```python
from build123d import *

# Parameters (mm, degrees)
RESSALTO_EXTRUS_O1_DEPTH = 10


with BuildPart() as part:
    # Esboço1 → Ressalto-extrusão1 (new body)
    with BuildSketch(Plane.XY):
        with BuildLine():
            Line((0, 14), (0, 20))
            Line((0, 20), (0, 40))
            ThreePointArc((0, 40), (-2.5, 42.5), (-5, 40))
            Line((-5, 40), (-4.923076923, 39.384615385))
            Line((-4.923076923, 39.384615385), (-3.069859681, 24.558877449))
            ThreePointArc((-3.069859681, 24.558877449), (-23.734852986, -7.015643501), (10.775337309, -22.281261317))
            Line((10.775337309, -22.281261317), (6.095140296, -12.603541755))
            ThreePointArc((6.095140296, -12.603541755), (-13.646420494, -3.126532858), (0, 14))
        make_face()
    extrude(amount=RESSALTO_EXTRUS_O1_DEPTH)


solid = part.part
```
Model file for the job. Use its own axes, mm. Coordinates: 2 decimals unless noted, no trailing zeros. Order: outer loops, then holes, each group sorted by start corner. A loop starts at its lowest first (then second) coordinate and runs counter-clockwise, first axis right, second up. Notation, with made-up numbers: (-23.5, -32.5) -> (13.5, -32.5) arc R11 ccw to (13.5, -18.5) -> close; hole circle Ø7 at (36, 35). An arc over 180 degrees is marked (long way). Answer as a JSON object with one key per item and string values. Group by question number.
1) Pull direction X, two halves, no side cores. Call faces 1 (the face through (-23.898, -6.437, 4.93)), 2 (the face through (-13.564, -3.469, 4.93)), 3 (the face through (-15, -1, 10)), 4 (the face through (0, 27, 5)): +X half, -X half, draft (parallel to the pull), parting line (faces both ways), or undercut.
2) Flat gauge pins, fed straight in: pin 1 (2 mm diameter, centred on y = 25.5, z = 2, fed in from +X); pin 2 (17 mm diameter, centred on x = 0, y = 0, fed in from -Z); pin 3 (2 mm diameter, centred on x = 6, z = 3, fed in from +Y). Where does each tip first touch, or does it go through?
3) Drill centre lines: L1, parallel to Y at x = -10, z = 4; L2, parallel to Y at x = -8.5, z = 1.75; L3, parallel to X at y = 0, z = 3.5. Where is each one in solid material? Low to high.
4) Cut at B-B, the plane z = 1. Write the cut outline in (x, y).
5) Cut at C-C, the plane y = 0. Write the cut outline in (x, z), then the cut area to 4 significant figures.
6) Cut at A-A, the plane x = -11. Write the cut outline in (y, z), then the cut area to 3 significant figures.
7) Cut at D-D, the plane y = 26.5. Write the cut outline in (x, z), then the cut area to 3 significant figures.
Check values:
{
 "1": {"face 1": "parting line", "face 2": "undercut", "face 3": "draft", "face 4": "+X half"},
 "2": {"pin 1": "stops at x = 0", "pin 2": "passes through", "pin 3": "stops at y = -12.6"},
 "3": {"L1": "y = -22.64 to -9.8, 9.8 to 22.64", "L2": "y = -23.24 to -11.12, 11.12 to 23.24", "L3": "x = -24.75 to -14"},
 "4": {"outline": "(-5, 40) -> (-3.07, 24.56) arc R24.75 ccw (long way) to (10.78, -22.28) -> (6.1, -12.6) arc R14 cw (long way) to (0, 14) -> (0, 40) arc R2.5 ccw to start"},
 "5": {"outline": "(-24.75, 0) -> (-14, 0) -> (-14, 10) -> (-24.75, 10) -> close", "area": "107.5 mm²"},
 "6": {"outline": "(-22.17, 0) -> (-8.66, 0) -> (-8.66, 10) -> (-22.17, 10) -> close; (8.66, 0) -> (22.17, 0) -> (22.17, 10) -> (8.66, 10) -> close", "area": "270 mm²"},
 "7": {"outline": "(-3.31, 0) -> (0, 0) -> (0, 10) -> (-3.31, 10) -> close", "area": "33.1 mm²"}
}
